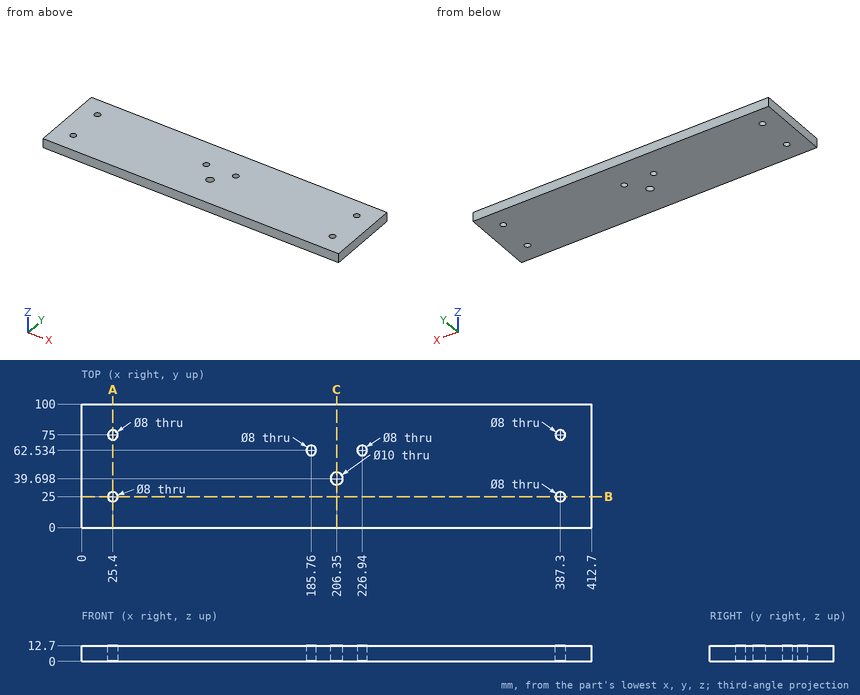
Could you check a few things on this drawing? It's one solid part, dimensions in mm from its lowest x, y, z. Round coordinates to 2 decimals unless told otherwise and drop trailing zeros. Order: outer loops, then holes, each group sorted by start corner. A loop starts at its lowest first (then second) coordinate and runs counter-clockwise, first axis right, second up.
Q1. Imagine slicing it at C-C, the plane x = 206.35. List the corners of the cut face in (y, z) for me, then the cut area to 3 significant figures.
Geometry says:
outline: (0, 0) - (34.7, 0) - (34.7, 12.7) - (0, 12.7) - close; (44.7, 0) - (100, 0) - (100, 12.7) - (44.7, 12.7) - close
area: 1,140 mm2
Q2. Imagine slicing it at A-A, the plane x = 25.4. List the corners of the cut face in (y, z) for me, then the cut area to 3 significant figures.
Geometry says:
outline: (0, 0) - (21, 0) - (21, 12.7) - (0, 12.7) - close; (29, 0) - (71, 0) - (71, 12.7) - (29, 12.7) - close; (79, 0) - (100, 0) - (100, 12.7) - (79, 12.7) - close
area: 1,070 mm2
Q3. Please list where these lines run through material, in increasing order: probe 1 along Y at (x, z) = (387.3, 4); probe 2 along X at (y, z) = (39.5, 2.25) (1 decimal); probe 3 along X at (y, z) = (42.5, 9.5).
Geometry says:
probe 1: y = 0 to 21, 29 to 71, 79 to 100
probe 2: x = 0 to 201.4, 211.3 to 412.7
probe 3: x = 0 to 202.21, 210.49 to 412.7
Q4. Imagine slicing it at B-B, the plane y = 25. List the corners of the cut face in (x, z) for me.
Geometry says:
outline: (0, 0) - (21.4, 0) - (21.4, 12.7) - (0, 12.7) - close; (29.4, 0) - (383.3, 0) - (383.3, 12.7) - (29.4, 12.7) - close; (391.3, 0) - (412.7, 0) - (412.7, 12.7) - (391.3, 12.7) - close
Q5. I'm going to push a flat-ended pin straight in: P1, Ø13, axis at x = 206.35, y = 39.7, coming from the +Z side. Where does the tip first touch, or does it pass through?
Geometry says:
P1: stops at z = 12.7
